Here's how the part is built. I have some questions about the finished solid (model axes, mm). A direction names the side the tool comes from. Round coordinates to 2 decimals unless told otherwise and drop trailing zeros. Use one line per item in the form item = value. Start each with the question number.
Q1. For faces 1 (the face through (0, -112, 0)), 2 (the face through (0.4, 807.5, 0)), 3 (the face through (0, 625, 9.525)), which set-ups out of +Z, -Z, +X, -X, +Y, -Y let a thin tool reach every point of the face, with its end or its side?
Q2. I'm going to push flat-ended pins straight in: pin 1 Ø1.4 at (x, z) = (1.5, 1.5) entering from -Y; pin 2 Ø15 at (x, y) = (-10.5, 2110.5) entering from +Z; pin 3 Ø1 at (x, z) = (-15, -6) entering from -Y (3 decimals). Where does each tip first touch, or does it pass through?
Q3. I need wall thicknesses on line 1 along Y through (x, z) = (6, 4.5); line 2 along Y through (x, z) = (1, 3) (3 decimals); line 3 along Y through (x, z) = (0, -3.25) (1 decimal). Which ranges of each line are inside material? Lowest first, please. Write a range as from..to.
Q4. We'd pull the mould along Y, two halves only. Please class faces 4 (the face through (0, 984, -9.525)), 5 (the face through (0, 1682, 0)): +Y half, -Y half, draft (parallel to the pull), parting line (faces both ways), or undercut.
```python
from build123d import *

# Parameters (mm, degrees)
F1_DEPTH = 25.4
F3_R     = 4.7625
F4_DEPTH = 9.525
F5_R     = 4.7625
F6_DEPTH = 25.4


with BuildPart() as f1:
    # F0 (on Right) → F1 (new body, symmetric)
    with BuildSketch(Plane.YZ):
        Polygon((-33.290768, -9.525), (2133.6, -9.525), (2133.6, 0), (2082.8, 0), (2082.8, 9.525), (1701.8, 9.525), (1701.8, 0), (1651, 0), (1651, 9.525), (838.2, 9.525), (838.2, 0), (787.4, 0), (787.4, 9.525), (457.2, 9.525), (457.2, 0), (406.4, 0), (406.4, 9.525), (0, 9.525), (-82.55, 9.525), (-82.55, 0), (-142.875, 0), (-133.35, -9.525), align=None)
    extrude(amount=F1_DEPTH, both=True)

    # F3 (on offset) → F4 (join)
    with BuildSketch(Plane.XZ.offset(-2133.6)):
        Circle(F3_R)
    extrude(amount=-F4_DEPTH)

    # F5 (on Top) → F6 (cut)
    with BuildSketch(Plane.XY):
        with Locations((0, 447.675)):
            Circle(F5_R)
        with Locations((0, 812.8)):
            Circle(F5_R)
        with Locations((0, 1676.4)):
            Circle(F5_R)
        with Locations((0, 2124.075)):
            Circle(F5_R)
    extrude(amount=-F6_DEPTH, mode=Mode.SUBTRACT)


solid = f1.part
```
Reported:
q1.face_1 = +Z, +X, -X, -Y
q1.face_2 = +Z, +X, -X
q1.face_3 = +Z, +X, -X, +Y, -Y
q2.pin_1 = -82.55
q2.pin_2 = 0
q2.pin_3 = -137.375
q3.line_1 = -82.55..406.4, 457.2..787.4, 838.2..1651, 1701.8..2082.8
q3.line_2 = -82.55..406.4, 457.2..787.4, 838.2..1651, 1701.8..2082.8, 2133.6..2143.125
q3.line_3 = -139.6..442.9, 452.4..808, 817.6..1671.6, 1681.2..2119.3, 2128.8..2143.1
q4.face_4 = draft
q4.face_5 = undercut
